Part model, mm, in its own coordinate system. Give positions to 0.01 mm unless a question says otherwise; leave off trailing zeros. Order: outer loops, then holes, each group sorted by start corner. A loop starts at its lowest first (then second) coordinate and runs counter-clockwise, first axis right, second up. Notation, with made-up numbers: (26, -18) -> (48, -18) arc R14 cw to (48, 3) -> close; hole circle Ø8 at (73.25, 85). An arc over 180 degrees is marked (long way). Write item = value, one per line. Start each with the question number.
Item 1: Band-saw the part on C-C on x = 4. Write the cut outline in (y, z).
Item 2: Flat gauge pins, fed straight in: P1, Ø1, axis at x = -112, y = -141, coming from the -Z side; P2, Ø6, axis at y = -145.5, z = 1718.5, coming from the +X side. Where does each tip first touch, or does it go through?
Item 3: Band-saw the part on A-A on z = 921. Write the cut outline in (x, y), plus the area to 3 significant figures.
Item 4: Drill centre lines: line 1 along X through (y, z) = (-143, 1997.5); line 2 along X through (y, z) = (-141.25, 1264.5); line 3 along Z through (x, y) = (293.5, -142). Where is each one in solid material? Low to high.
Item 5: Band-saw the part on B-B on y = -144. Write the cut outline in (x, z).
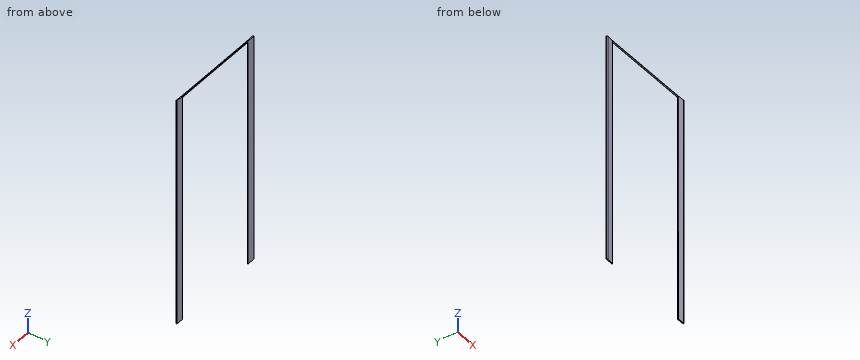
```python
from build123d import *

# Parameters (mm, degrees)
SKETCH278_W         = 1600
SKETCH278_H         = 400
EXTRUDE039512_DEPTH = 500


with BuildPart() as extrude039512:
    # Sketch278 (on Sketch) → Extrude039512 (new body, symmetric)
    with BuildSketch(Plane.XZ):
        with Locations((0, 2300)):
            Rectangle(SKETCH278_W, SKETCH278_H)
        with Locations((0, -200)):
            Rectangle(SKETCH278_W, SKETCH278_H)
    extrude(amount=EXTRUDE039512_DEPTH, both=True)


with BuildPart() as trim_two_parts_external:
    # Sweep011: sweep along a path in Sketch194
    with BuildLine(Plane.XZ.offset(140)) as sweep011_path:
        Line((-390, 2090), (-390, 0))
        Line((-390, 0), (390, 0))
        Line((390, 0), (390, 2090))
        Line((390, 2090), (-390, 2090))
    # Clone2D027 (on Sketch) → Sweep011 (sweep)
    with BuildSketch(Plane(origin=(0, -140, 0), x_dir=(0, 0, 1), z_dir=(1, 0, 0))):
        with BuildLine():
            Line((-61.571224, 10), (-5.678418, 7))
            ThreePointArc((-5.678418, 7), (-1.645147, 5.136003), (0, 1.008624))
            Line((0, 1.008624), (0, 0))
            Line((0, 0), (-70, 0))
            Line((-70, 0), (-70, 2.011499))
            ThreePointArc((-70, 2.011499), (-67.503171, 7.81797), (-61.571224, 10))
        make_face()
    sweep(path=sweep011_path.line, is_frenet=True, transition=Transition.RIGHT)

    # Cut077: cut Extrude039512
    add(extrude039512.part, mode=Mode.SUBTRACT)


solid = trim_two_parts_external.part
```
Values found:
q1.outline = (-147.23, 2100) -> (-147, 2095.68) arc R6 ccw to (-141.01, 2090) -> (-140, 2090) -> (-140, 2100) -> close
q2.P1 = 2090
q2.P2 = 459.99
q3.outline = (-460, -142.01) arc R8 ccw to (-451.57, -150) -> (-395.68, -147) arc R6 ccw to (-390, -141.01) -> (-390, -140) -> (-460, -140) -> close; (390, -141.01) arc R6 ccw to (395.68, -147) -> (451.57, -150) arc R8 ccw to (460, -142.01) -> (460, -140) -> (390, -140) -> close
q3.area = 1,160 mm^2
q4.line_1 = -459.94 to -390.34, 390.34 to 459.94
q4.line_2 = -460 to -390, 390 to 460
q4.line_3 = 2090.08 to 2100
q5.outline = (-459.75, 0) -> (-390.8, 0) -> (-390.8, 2090.8) -> (390.8, 2090.8) -> (390.8, 0) -> (459.75, 0) -> (459.75, 2100) -> (-459.75, 2100) -> close
